Read the model definition and answer for the solid it produces. Units are mm, in the model's axes. Face numbers are marked on the shaded views. A direction names the side the tool comes from. Coordinates: 2 decimals unless noted, no trailing zeros. Order: outer loops, then holes, each group sorted by start corner. A loop starts at its lowest first (then second) coordinate and runs counter-clockwise, first axis right, second up. Notation, with made-up numbers: (17, 9) -> (73, 9) arc R11 cw to (73, 14) -> close; hole circle Ø5 at (35.25, 32.5). An arc over 180 degrees is marked (long way). Return JSON: item names as keys, results as strings. Group by question number.
Autodesk Inventor part; units mm, degrees
ref_plane "YZ Plane" through (0, 0, 0) normal (1, 0, 0) x (0, 1, 0)
ref_plane "XZ Plane" through (0, 0, 0) normal (0, 1, 0) x (-1, 0, 0)
ref_plane "XY Plane" through (0, 0, 0) normal (0, 0, 1) x (1, 0, 0)
sketch "Sketch1" plane through (0, 0, 0) normal (0, 1, 0) x (-1, 0, 0)
  line L0 (-100, 100) -> (100, 100)
  line L1 (100, 100) -> (100, -100)
  line L2 (100, -100) -> (-100, -100)
  line L3 (-100, -100) -> (-100, 100)
  line L4 (-100, 100) -> (100, -100) construction
  line L5 (100, 100) -> (-100, -100) construction
  line L6 (103.175, -103.175) -> (103.175, 103.175)
  line L7 (103.175, 103.175) -> (-103.175, 103.175)
  line L8 (-103.175, 103.175) -> (-103.175, -103.175)
  line L9 (-103.175, -103.175) -> (103.175, -103.175)
  point P0 (0, 0)
  dimension "d0" = 200
  dimension "d1" = 3.175
extrude "Extrusion1" add sketch "Sketch1" along normal blind 410
sketch "Sketch2" plane through (0, 410, 0) normal (0, 1, 0) x (1, 0, 0)
  line L0 (-100, -100) -> (-100, 100)
  line L1 (-100, 100) -> (100, 100)
  line L2 (100, 100) -> (100, -100)
  line L3 (100, -100) -> (-100, -100)
  line L4 (-103.175, 103.175) -> (-103.175, -103.175)
  line L5 (-103.175, -103.175) -> (103.175, -103.175)
  line L6 (103.175, -103.175) -> (103.175, 103.175)
  line L7 (103.175, 103.175) -> (-103.175, 103.175)
  point P0 (0, 0)
extrude "Extrusion2" add sketch "Sketch2" along normal blind 3.175 contours L0 L1 L2 L3 | L7 L6 L5 L4
sketch "Sketch3" plane through (103.175, 0, 103.175) normal (1, 0, 0) x (0, 0, -1)
  line L0 (0, 0) -> (206.35, 0)
  line L1 (206.35, 0) -> (206.35, 413.175)
  line L2 (0, 413.175) -> (206.35, 413.175)
  line L3 (0, 0) -> (0, 413.175)
  line L4 (206.35, 0) -> (0, 0)
  line L5 (186.35, 0) -> (186.35, 50)
  line L6 (186.35, 50) -> (20, 50)
  line L7 (20, 50) -> (20, 0)
  line L8 (20, 263.175) -> (20, 143.175)
  line L9 (20, 143.175) -> (186.35, 143.175)
  line L10 (186.35, 143.175) -> (186.35, 263.175)
  line L11 (186.35, 263.175) -> (20, 263.175)
  point P0 (103.175, 0)
  dimension "d6" = 50
  dimension "d7" = 20
  dimension "d8" = 20
  dimension "d9" = 150
  dimension "d12" = 120
extrude "Extrusion3" cut sketch "Sketch3" against normal up to surface (206.35 mm away) contours L7 L6 L5 L0 | L11 L10 L9 L8
properties part number "Cover"
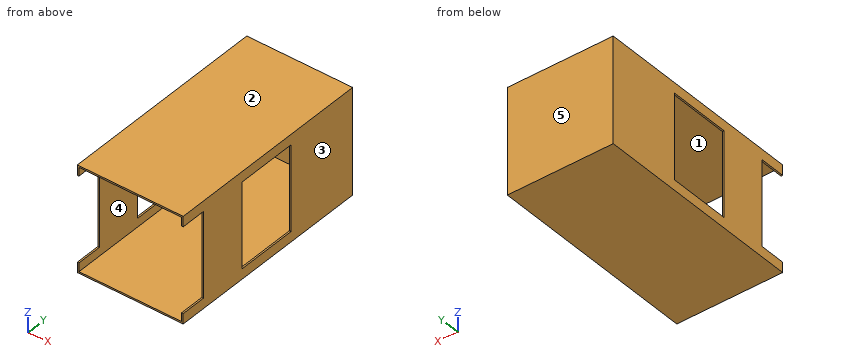
1. Which of the six approach directions +Z, -Z, +X, -X, +Y, -Y give full straight-line access (tool end or side, diameter ignored) to the marked faces 4 and 5?
2. Find section B-B on y = 375. Determine the outline of the cut face in (x, z) (3 decimals).
3. For a pull along X with two mould halves and no side action, classify the marked faces 1, 2 and 3 as released by +X, released by -X, zero draft, split by the parting line, or undercut.
4. Straight lines are drawn through the part: L1, parallel to Z at x = 71, y = 119 (3 decimals); L2, parallel to Y at x = 38, z = -78 (3 decimals). For each, find the intervals that lie inside material, in ascending order.
5. Find section C-C on x = -45.5. Determine the outline of the cut face in (y, z) (3 decimals).
6. Find section D-D on z = -89. Determine the outline of the cut face in (x, y) (3 decimals), and give its area (3 significant figures).
7. Given pin 1 (3.5 mm diameter, centred on x = -102, z = -34.5, fed in from -Y); pin 2 (4 mm diameter, centred on x = -68, z = -50, fed in from -Y), each flat-ended and moving along its own axis, determine where each tip first touches the part or whether it passes through.
8. Find section A-A on z = -21.5. Determine the outline of the cut face in (x, y) (3 decimals), and give its area (3 significant figures).
Result:
{
 "1": {"face 4": "-Y", "face 5": "+Z, -Z, +X, -X, +Y"},
 "2": {"outline": "(-103.175, -103.175) -> (103.175, -103.175) -> (103.175, 103.175) -> (-103.175, 103.175) -> close; hole (-100, -100) -> (100, -100) -> (100, 100) -> (-100, 100) -> close"},
 "3": {"face 1": "undercut", "face 2": "zero draft", "face 3": "released by +X"},
 "4": {"L1": "-103.175 to -100, 100 to 103.175", "L2": "410 to 413.175"},
 "5": {"outline": "(0, -103.175) -> (413.175, -103.175) -> (413.175, 103.175) -> (0, 103.175) -> (0, 100) -> (410, 100) -> (410, -100) -> (0, -100) -> close"},
 "6": {"outline": "(-103.175, 0) -> (-100, 0) -> (-100, 410) -> (100, 410) -> (100, 0) -> (103.175, 0) -> (103.175, 413.175) -> (-103.175, 413.175) -> close", "area": "3,260 mm^2"},
 "7": {"pin 1": "y = 50", "pin 2": "y = 410"},
 "8": {"outline": "(-103.175, 50) -> (-100, 50) -> (-100, 143.175) -> (-103.175, 143.175) -> close; (-103.175, 263.175) -> (-100, 263.175) -> (-100, 410) -> (100, 410) -> (100, 263.175) -> (103.175, 263.175) -> (103.175, 413.175) -> (-103.175, 413.175) -> close; (100, 50) -> (103.175, 50) -> (103.175, 143.175) -> (100, 143.175) -> close", "area": "2,180 mm^2"}
}
